from build123d import *
from build123d.topology import SkipClean

# Parameters (mm, degrees)
SKETCH1_R           = 2.5
SKETCH1_R_2         = 15
SKETCH1_R_3         = 17.5
SKETCH1_R_4         = 20
SKETCH1_R_5         = 10
SKETCH1_R_6         = 12.5
BOSS_EXTRUDE2_DEPTH = 5
SKETCH1_5_R         = 2.5
BOSS_EXTRUDE3_DEPTH = 32.5
SKETCH1_6_R         = 2.5
CUT_EXTRUDE1_DEPTH  = 25
BOSS_EXTRUDE4_START = -10
SKETCH1_7_R         = 17.5
SKETCH1_7_R_2       = 12.5
SKETCH1_7_R_3       = 20
SKETCH1_7_R_4       = 15
BOSS_EXTRUDE4_DEPTH = 10
CUT_EXTRUDE2_START  = -5
SKETCH1_8_R         = 12.5
SKETCH1_8_R_2       = 15
CUT_EXTRUDE2_DEPTH  = 5
SKETCH1_9_R         = 15
SKETCH1_9_R_2       = 10
BOSS_EXTRUDE5_DEPTH = 10
SKETCH1_10_R        = 10
CUT_EXTRUDE4_DEPTH  = 5
CUT_EXTRUDE5_START  = -10
SKETCH1_11_R        = 15
CUT_EXTRUDE5_DEPTH  = 10
SKETCH1_12_R        = 2.5
BOSS_EXTRUDE7_DEPTH = 32.5
SKETCH1_14_R        = 2.5
CUT_EXTRUDE7_DEPTH  = 25


with BuildPart() as part:
    # Sketch1 → Boss-Extrude2 (new body)
    # profile 1 of 6: a face of its own
    with BuildSketch(Plane.XY):
        with BuildLine():
            ThreePointArc((-105.836575371, -69.405122728), (-101.525256537, -68.223407914), (-97.905442155, -65.600267844))
            ThreePointArc((-97.905442155, -65.600267844), (-73.850667048, -67.721382917), (-50.571382583, -61.302173509))
            ThreePointArc((-50.571382583, -61.302173509), (-43.775658453, -63.659612747), (-36.80587195, -61.881562601))
            ThreePointArc((-36.80587195, -61.881562601), (72, 0), (-36.80587195, 61.881562601))
            ThreePointArc((-36.80587195, 61.881562601), (-43.775658453, 63.659612747), (-50.571382583, 61.302173509))
            ThreePointArc((-50.571382583, 61.302173509), (-123.538014062, 52.234484122), (-145.600267844, -17.905442155))
            ThreePointArc((-145.600267844, -17.905442155), (-148.223407914, -21.525256537), (-149.405122728, -25.836575371))
            ThreePointArc((-149.405122728, -25.836575371), (-156.367532368, -76.367532368), (-105.836575371, -69.405122728))
        make_face()
        with Locations((-143.85414855, -23.38049856)):
            Circle(SKETCH1_R, mode=Mode.SUBTRACT)
        with Locations((-43.5, 57.373774497)):
            Circle(SKETCH1_R, mode=Mode.SUBTRACT)
        with Locations((-103.38049856, -63.85414855)):
            Circle(SKETCH1_R, mode=Mode.SUBTRACT)
        with Locations((-43.5, -57.373774497)):
            Circle(SKETCH1_R, mode=Mode.SUBTRACT)
        with BuildLine():
            ThreePointArc((-106.931982072, -56.953211864), (-74.302823883, -62.741869468), (-43.25, -51.17067031))
            ThreePointArc((-43.25, -51.17067031), (67, 0), (-43.25, 51.17067031))
            ThreePointArc((-43.25, 51.17067031), (-120.336689499, 48.393713231), (-136.953211864, -26.931982072))
            ThreePointArc((-136.953211864, -26.931982072), (-152.831998462, -72.831998462), (-106.931982072, -56.953211864))
        make_face(mode=Mode.SUBTRACT)
    # profile 2 of 6: a face of its own
    with BuildSketch(Plane.XY):
        with BuildLine():
            ThreePointArc((-136.953211864, -26.931982072), (-152.831998462, -72.831998462), (-106.931982072, -56.953211864))
            ThreePointArc((-106.931982072, -56.953211864), (-74.302823883, -62.741869468), (-43.25, -51.17067031))
            ThreePointArc((-43.25, -51.17067031), (67, 0), (-43.25, 51.17067031))
            ThreePointArc((-43.25, 51.17067031), (-120.336689499, 48.393713231), (-136.953211864, -26.931982072))
        make_face()
        with Locations((-133.74011537, -53.74011537)):
            Circle(SKETCH1_R_2, mode=Mode.SUBTRACT)
        with Locations((-80, 0)):
            Circle(SKETCH1_R_3, mode=Mode.SUBTRACT)
        Circle(SKETCH1_R_4, mode=Mode.SUBTRACT)
    # profile 3 of 6: a face of its own
    with BuildSketch(Plane.XY):
        with Locations((-133.74011537, -53.74011537)):
            Circle(SKETCH1_R_2)
        with Locations((-133.74011537, -53.74011537)):
            Circle(SKETCH1_R_5, mode=Mode.SUBTRACT)
    # profile 4 of 6: a face of its own
    with BuildSketch(Plane.XY):
        with Locations((-133.74011537, -53.74011537)):
            Circle(SKETCH1_R_5)
    # profile 5 of 6: a face of its own
    with BuildSketch(Plane.XY):
        with Locations((-80, 0)):
            Circle(SKETCH1_R_3)
        with Locations((-80, 0)):
            Circle(SKETCH1_R_6, mode=Mode.SUBTRACT)
    # profile 6 of 6: a face of its own
    with BuildSketch(Plane.XY):
        Circle(SKETCH1_R_4)
        Circle(SKETCH1_R_2, mode=Mode.SUBTRACT)
    extrude(amount=BOSS_EXTRUDE2_DEPTH)

    # Sketch1_5 → Boss-Extrude3 (add)
    # profile 1 of 2: a face of its own
    with BuildSketch(Plane.XY):
        with BuildLine():
            ThreePointArc((-105.836575371, -69.405122728), (-101.525256537, -68.223407914), (-97.905442155, -65.600267844))
            ThreePointArc((-97.905442155, -65.600267844), (-73.850667048, -67.721382917), (-50.571382583, -61.302173509))
            ThreePointArc((-50.571382583, -61.302173509), (-43.775658453, -63.659612747), (-36.80587195, -61.881562601))
            ThreePointArc((-36.80587195, -61.881562601), (72, 0), (-36.80587195, 61.881562601))
            ThreePointArc((-36.80587195, 61.881562601), (-43.775658453, 63.659612747), (-50.571382583, 61.302173509))
            ThreePointArc((-50.571382583, 61.302173509), (-123.538014062, 52.234484122), (-145.600267844, -17.905442155))
            ThreePointArc((-145.600267844, -17.905442155), (-148.223407914, -21.525256537), (-149.405122728, -25.836575371))
            ThreePointArc((-149.405122728, -25.836575371), (-156.367532368, -76.367532368), (-105.836575371, -69.405122728))
        make_face()
        with Locations((-143.85414855, -23.38049856)):
            Circle(SKETCH1_5_R, mode=Mode.SUBTRACT)
        with Locations((-43.5, 57.373774497)):
            Circle(SKETCH1_5_R, mode=Mode.SUBTRACT)
        with Locations((-103.38049856, -63.85414855)):
            Circle(SKETCH1_5_R, mode=Mode.SUBTRACT)
        with Locations((-43.5, -57.373774497)):
            Circle(SKETCH1_5_R, mode=Mode.SUBTRACT)
        with BuildLine():
            ThreePointArc((-106.931982072, -56.953211864), (-74.302823883, -62.741869468), (-43.25, -51.17067031))
            ThreePointArc((-43.25, -51.17067031), (67, 0), (-43.25, 51.17067031))
            ThreePointArc((-43.25, 51.17067031), (-120.336689499, 48.393713231), (-136.953211864, -26.931982072))
            ThreePointArc((-136.953211864, -26.931982072), (-152.831998462, -72.831998462), (-106.931982072, -56.953211864))
        make_face(mode=Mode.SUBTRACT)
    # profile 2 of 2: a face of its own
    with BuildSketch(Plane.XY):
        with BuildLine():
            Line((92, -15), (92, 0))
            Line((92, 0), (92, 15))
            ThreePointArc((92, 15), (90.535533906, 18.535533906), (87, 20))
            Line((87, 20), (69.166465863, 20))
            ThreePointArc((69.166465863, 20), (72, 0), (69.166465863, -20))
            Line((69.166465863, -20), (87, -20))
            ThreePointArc((87, -20), (90.535533906, -18.535533906), (92, -15))
        make_face()
        with Locations((82, -10)):
            Circle(SKETCH1_5_R, mode=Mode.SUBTRACT)
        with Locations((82, 10)):
            Circle(SKETCH1_5_R, mode=Mode.SUBTRACT)
    extrude(amount=BOSS_EXTRUDE3_DEPTH)

    # Sketch1_6 → Cut-Extrude1 (cut)
    with SkipClean():  # the faces are left unmerged after this step: merging them gives an invalid solid
        with BuildSketch(Plane.XY):
            with BuildLine():
                Line((92, -15), (92, 0))
                Line((92, 0), (92, 15))
                ThreePointArc((92, 15), (90.535533906, 18.535533906), (87, 20))
                Line((87, 20), (69.166465863, 20))
                ThreePointArc((69.166465863, 20), (72, 0), (69.166465863, -20))
                Line((69.166465863, -20), (87, -20))
                ThreePointArc((87, -20), (90.535533906, -18.535533906), (92, -15))
            make_face()
            with Locations((82, -10)):
                Circle(SKETCH1_6_R, mode=Mode.SUBTRACT)
            with Locations((82, 10)):
                Circle(SKETCH1_6_R, mode=Mode.SUBTRACT)
        extrude(amount=CUT_EXTRUDE1_DEPTH, mode=Mode.SUBTRACT)

    # Sketch1_7 → Boss-Extrude4 (add)
    # profile 1 of 4: a face of its own
    with SkipClean():  # the faces are left unmerged after this step: merging them gives an invalid solid
        with BuildSketch(Plane.XY.offset(BOSS_EXTRUDE4_START)):
            with Locations((-80, 0)):
                Circle(SKETCH1_7_R)
            with Locations((-80, 0)):
                Circle(SKETCH1_7_R_2, mode=Mode.SUBTRACT)
        # profile 2 of 4: a face of its own
        with BuildSketch(Plane.XY.offset(BOSS_EXTRUDE4_START)):
            with Locations((-80, 0)):
                Circle(SKETCH1_7_R_2)
        # profile 3 of 4: a face of its own
        with BuildSketch(Plane.XY.offset(BOSS_EXTRUDE4_START)):
            Circle(SKETCH1_7_R_3)
            Circle(SKETCH1_7_R_4, mode=Mode.SUBTRACT)
        # profile 4 of 4: a face of its own
        with BuildSketch(Plane.XY.offset(BOSS_EXTRUDE4_START)):
            Circle(SKETCH1_7_R_4)
        extrude(amount=BOSS_EXTRUDE4_DEPTH)

    # Sketch1_8 → Cut-Extrude2 (cut)
    with SkipClean():  # the faces are left unmerged after this step: merging them gives an invalid solid
        with BuildSketch(Plane.XY.offset(CUT_EXTRUDE2_START)):
            with Locations((-80, 0)):
                Circle(SKETCH1_8_R)
            Circle(SKETCH1_8_R_2)
        extrude(amount=CUT_EXTRUDE2_DEPTH, mode=Mode.SUBTRACT)

    # Sketch1_9 → Boss-Extrude5 (add)
    with SkipClean():  # the faces are left unmerged after this step: merging them gives an invalid solid
        with BuildSketch(Plane.XY):
            with Locations((-133.74011537, -53.74011537)):
                Circle(SKETCH1_9_R)
            with Locations((-133.74011537, -53.74011537)):
                Circle(SKETCH1_9_R_2, mode=Mode.SUBTRACT)
        extrude(amount=-BOSS_EXTRUDE5_DEPTH)

    # Sketch1_10 → Cut-Extrude4 (cut, symmetric)
    with SkipClean():  # the faces are left unmerged after this step: merging them gives an invalid solid
        with BuildSketch(Plane.XY):
            with Locations((-133.74011537, -53.74011537)):
                Circle(SKETCH1_10_R)
        extrude(amount=CUT_EXTRUDE4_DEPTH, both=True, mode=Mode.SUBTRACT)

    # Sketch1_11 → Cut-Extrude5 (cut)
    with SkipClean():  # the faces are left unmerged after this step: merging them gives an invalid solid
        with BuildSketch(Plane.XY.offset(CUT_EXTRUDE5_START)):
            Circle(SKETCH1_11_R)
        extrude(amount=CUT_EXTRUDE5_DEPTH, mode=Mode.SUBTRACT)

    # Sketch1_12 → Boss-Extrude7 (add)
    with SkipClean():  # the faces are left unmerged after this step: merging them gives an invalid solid
        with BuildSketch(Plane.XY):
            with BuildLine():
                ThreePointArc((-147.07619641, 11.17067031), (-139.39821809, 33.103650671), (-124.783507009, 51.17067031))
                Line((-124.783507009, 51.17067031), (-143.891753504, 51.17067031))
                Line((-143.891753504, 51.17067031), (-163, 51.17067031))
                ThreePointArc((-163, 51.17067031), (-166.535533906, 49.706204216), (-168, 46.17067031))
                Line((-168, 46.17067031), (-168, 16.17067031))
                ThreePointArc((-168, 16.17067031), (-166.535533906, 12.635136404), (-163, 11.17067031))
                Line((-163, 11.17067031), (-147.07619641, 11.17067031))
            make_face()
            with Locations((-154, 25.585335155)):
                Circle(SKETCH1_12_R, mode=Mode.SUBTRACT)
            with Locations((-154, 38.378002733)):
                Circle(SKETCH1_12_R, mode=Mode.SUBTRACT)
        extrude(amount=BOSS_EXTRUDE7_DEPTH)

    # Sketch1_14 → Cut-Extrude7 (cut)
    with SkipClean():  # the faces are left unmerged after this step: merging them gives an invalid solid
        with BuildSketch(Plane.XY):
            with BuildLine():
                ThreePointArc((-147.07619641, 11.17067031), (-139.39821809, 33.103650671), (-124.783507009, 51.17067031))
                Line((-124.783507009, 51.17067031), (-143.891753504, 51.17067031))
                Line((-143.891753504, 51.17067031), (-163, 51.17067031))
                ThreePointArc((-163, 51.17067031), (-166.535533906, 49.706204216), (-168, 46.17067031))
                Line((-168, 46.17067031), (-168, 16.17067031))
                ThreePointArc((-168, 16.17067031), (-166.535533906, 12.635136404), (-163, 11.17067031))
                Line((-163, 11.17067031), (-147.07619641, 11.17067031))
            make_face()
            with Locations((-154, 25.585335155)):
                Circle(SKETCH1_14_R, mode=Mode.SUBTRACT)
            with Locations((-154, 38.378002733)):
                Circle(SKETCH1_14_R, mode=Mode.SUBTRACT)
        extrude(amount=CUT_EXTRUDE7_DEPTH, mode=Mode.SUBTRACT)


solid = part.part
The model under review builds one solid part; all positions refer to its coordinate system, in mm. A direction names the side the tool comes from. Give positions to 0.01 mm unless a question says otherwise; leave off trailing zeros. Write each loop counter-clockwise with the first axis right and the second up, starting at its lowest first coordinate (ties: lowest second). Pieces come first, ordered by that corner, then holes.
1. Add section A-A, the plane y = 0. Write out the cut boundary in (x, z).
2. Add section B-B, the plane x = -80. Write out the cut boundary in (y, z).
3. Draft analysis for pull direction X (two halves, no side actions). For faces 5 (the cylindrical face through (-74.771, -62.783, 18.557)), 6 (the cylindrical face through (-148.196, -21.469, 16.022)), 7 (the cylindrical face through (90, -19, 29)), state which applies: +X half, -X half, draft (parallel to the pull), parting line (faces both ways), or undercut.
4. Wall thickness on L1, parallel to Y at x = 0, z = 11.5; L2, parallel to Y at x = -154, z = 29.25; L3, parallel to Y at x = -43, z = 19: over which ranges is each line inside the solid? List them lowest first.
5. Add section C-C, the plane x = -154. Write out the cut boundary in (y, z), plus the area to 3 significant figures.
6. Tool access review of faces 1 (the cylindrical face through (66.966, -2.131, 18.557)), 2 (the flat face through (-155, 11.171, 29)), 3 (the flat face through (78, 20, 29)), 4 (the flat face through (-49, -6, 0)): name each direction out of +Z, -Z, +X, -X, +Y, -Y from which nothing blocks a thin tool from reaching the whole face with its end or side.
7. For P1, Ø6, axis at x = -157.5, z = 28, coming from the -Y side; P2, Ø3, axis at x = -143.85, y = -23.38, coming from the +Z side; P3, Ø6, axis at x = 56.5, z = 16.5, coming from the -Y side; P4, Ø3, axis at y = -67, z = 23, coming from the -X side, all flat-tipped, find the tip position at first contact; note any pin that passes through.
8. Add section D-D, the plane z = 28.5. Count the separate pieces of the cut face and the enclosed holes in it, plus the area to 3 significant figures.
Worked answers:
1. outline: (-148, 0) - (-97.5, 0) - (-97.5, -10) - (-62.5, -10) - (-62.5, 0) - (-20, 0) - (-20, -10) - (-15, -10) - (-15, 5) - (-67.5, 5) - (-67.5, -5) - (-92.5, -5) - (-92.5, 5) - (-143, 5) - (-143, 32.5) - (-148, 32.5) - close; (15, -10) - (20, -10) - (20, 0) - (72, 0) - (72, 25) - (92, 25) - (92, 32.5) - (67, 32.5) - (67, 5) - (15, 5) - close
2. outline: (-68, 0) - (-17.5, 0) - (-17.5, -10) - (17.5, -10) - (17.5, 0) - (68, 0) - (68, 32.5) - (63, 32.5) - (63, 5) - (12.5, 5) - (12.5, -5) - (-12.5, -5) - (-12.5, 5) - (-63, 5) - (-63, 32.5) - (-68, 32.5) - close
3. face 5: undercut
3. face 6: -X half
3. face 7: +X half
4. L1: y = -72 to -67, 67 to 72
4. L2: y = -78.51 to -71.59, -35.89 to -28.97, 11.17 to 23.09, 28.09 to 35.88, 40.88 to 51.17
4. L3: y = -63.67 to -59.82, -54.92 to -51.38, 51.38 to 54.92, 59.82 to 63.67
5. outline: (-78.51, 0) - (-28.97, 0) - (-28.97, 32.5) - (-35.89, 32.5) - (-35.89, 5) - (-71.59, 5) - (-71.59, 32.5) - (-78.51, 32.5) - close; (11.17, 25) - (23.09, 25) - (23.09, 32.5) - (11.17, 32.5) - close; (28.09, 25) - (35.88, 25) - (35.88, 32.5) - (28.09, 32.5) - close; (40.88, 25) - (51.17, 25) - (51.17, 32.5) - (40.88, 32.5) - close
5. area: 853 mm2
6. face 1: +Z
6. face 2: +Z, -Z, -X
6. face 3: +Z, -Z, +X, +Y
6. face 4: -Z
7. P1: stops at y = -78.09
7. P2: passes through
7. P3: stops at y = -48.18
7. P4: stops at x = -163.5
8. separate pieces: 1
8. enclosed holes: 9
8. area: 5,300 mm2
